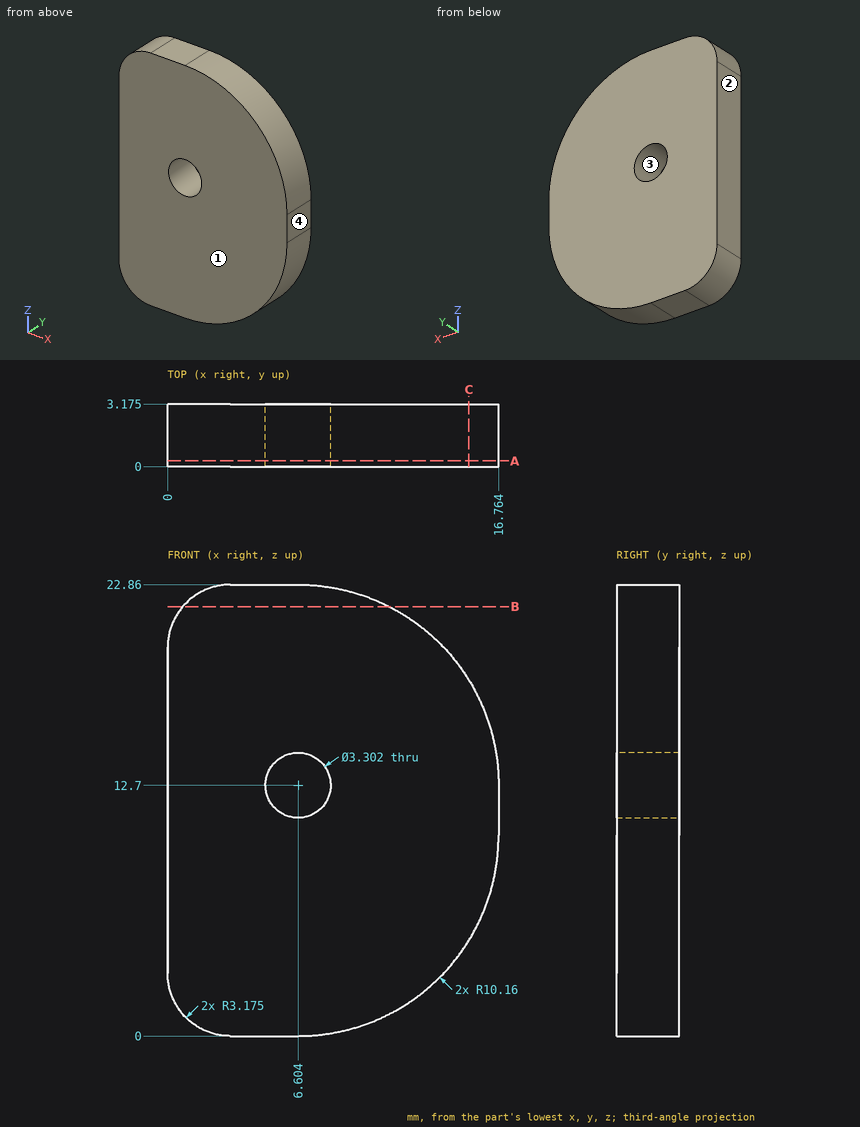
Geometry check sheet. Reference: drawing and pictorial views, mm from the part's lowest x, y, z. Coordinates: 2 decimals unless noted, no trailing zeros. Loops run counter-clockwise (first coordinate to the right, second up) from the corner with the lowest first, then second, coordinate; pieces in that order, holes last. Notation, with made-up numbers: (6, 35) - (45, 35) arc R20 ccw to (45, 43) - close; hole circle Ø1 at (62.25, 7.5). An arc over 180 degrees is marked (long way). Return JSON: item names as keys, results as strings.
1. Go/stop test with flat-tipped pins: pin 1 (1.5 mm diameter, centred on x = 8.5, y = 2.5, fed in from -Z); pin 2 (1 mm diameter, centred on x = 14.5, y = 0.5, fed in from +Z); pin 3 (1 mm diameter, centred on x = 10.5, z = 5.5, fed in from -Y). Record where each tip stops, or that it passes through.
Established:
{"pin 1": "stops at z = 0.06", "pin 2": "stops at z = 19.67", "pin 3": "stops at y = 0"}
2. Section check A-A, the plane y = 0.3. Record the boundary of the cut face in (x, z) (3 decimals), then the cut area to 3 significant figures.
Established:
{"outline": "(0, 3.175) arc R3.175 ccw to (3.175, 0) - (6.604, 0) arc R10.16 ccw to (16.764, 10.16) - (16.764, 12.7) arc R10.16 ccw to (6.604, 22.86) - (3.175, 22.86) arc R3.175 ccw to (0, 19.685) - close; hole circle Ø3.302 at (6.604, 12.7)", "area": "326 mm2"}
3. Section check B-B, the plane z = 21.75. Record the boundary of the cut face in (x, y) (3 decimals).
Established:
{"outline": "(0.763, 0) - (11.222, 0) - (11.222, 3.175) - (0.763, 3.175) - close"}
4. Section check C-C, the plane x = 15.25. Record the boundary of the cut face in (y, z) (3 decimals), then the cut area to 3 significant figures.
Established:
{"outline": "(0, 4.824) - (3.175, 4.824) - (3.175, 18.036) - (0, 18.036) - close", "area": "41.9 mm2"}
5. Thickness scan on L1, parallel to Z at x = 6.5, y = 2.45; L2, parallel to Z at x = 7.5, y = 0.6; L3, parallel to X at y = 1.55, z = 10. Record the ranges inside material, lowest first.
Established:
{"L1": "z = 0 to 11.05, 14.35 to 22.86", "L2": "z = 0.04 to 11.31, 14.09 to 22.82", "L3": "x = 0 to 16.76"}
6. Mould release check, pull along X, two halves, no side actions. Record for the marked faces 1, 2, 3 and 4: +X half, -X half, draft (parallel to the pull), parting line (faces both ways), or undercut.
Established:
{"face 1": "draft", "face 2": "-X half", "face 3": "undercut", "face 4": "+X half"}
